Build history of the part. All positions in model axes, mm. Face numbers are marked on the shaded views. A direction names the side the tool comes from. Round coordinates to 2 decimals unless told otherwise and drop trailing zeros. Order: outer loops, then holes, each group sorted by start corner. A loop starts at its lowest first (then second) coordinate and runs counter-clockwise, first axis right, second up. Notation, with made-up numbers: (69, 63) - (125, 63) arc R31 cw to (125, 92) - close; hole circle Ø4 at (40.25, -17.75). An arc over 180 degrees is marked (long way). One line per question, with ' | ' between items. Start each with the question number.
from build123d import *

# Parameters (mm, degrees)
SKETCH1_R          = 5
EXTRUDE1_DEPTH     = 40
SKETCH2_W          = 7
SKETCH2_H          = 34.499518557
SKETCH2_W_2        = 12
CUT_EXTRUDE1_DEPTH = 40


with BuildPart() as part:
    # Sketch1 → Extrude1 (new body)
    with BuildSketch(Plane.XY):
        with BuildLine():
            Line((15, -16), (25, -16))
            Line((25, -16), (25, -22))
            Line((25, -22), (-25, -22))
            Line((-25, -22), (-25, -16))
            Line((-25, -16), (-15, -16))
            Line((-15, -16), (-15, 0))
            ThreePointArc((-15, 0), (0, 15), (15, 0))
            Line((15, 0), (15, -16))
        make_face()
        Circle(SKETCH1_R, mode=Mode.SUBTRACT)
    extrude(amount=EXTRUDE1_DEPTH)

    # Sketch2 → Cut-Extrude1 (cut)
    with BuildSketch(Plane(origin=(15, 0, 0), x_dir=(0, 0, -1), z_dir=(1, 0, 0))):
        with Locations((-36.5, 1.249759279)):
            Rectangle(SKETCH2_W, SKETCH2_H)
        with Locations((-3.5, 1.249759279)):
            Rectangle(SKETCH2_W, SKETCH2_H)
        with Locations((-20, 1.249759279)):
            Rectangle(SKETCH2_W_2, SKETCH2_H)
    extrude(amount=-CUT_EXTRUDE1_DEPTH, mode=Mode.SUBTRACT)


solid = part.part
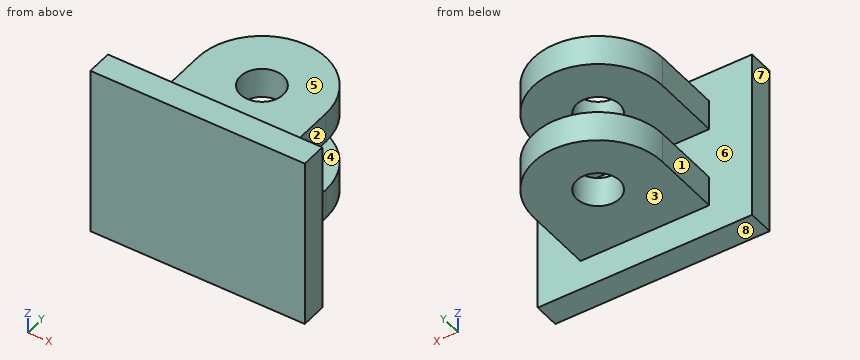
Item 1: Slice it at D-D (x = 6). Write the cut outline in (y, z).
Item 2: 3-axis set-ups, long thin cutter, end or side, ignore diameter. For the marked faces 1, 2, 3, 4 and 5: which of +Z, -Z, +X, -X, +Y, -Y reach the whole face in a straight line?
Item 3: Pull direction Z, two halves, no side cores. Call the marked faces 6, 7 and 8: released by +Z, released by -Z, zero draft, split by the parting line, or undercut.
Item 4: Pin check, flat tips, straight feed: pin 1 (9 mm diameter, centred on x = 4, y = 4, fed in from +Z); pin 2 (4 mm diameter, centred on x = 3, y = 8, fed in from -Z); pin 3 (3.5 mm diameter, centred on y = -9, z = 30, fed in from +X); pin 4 (6 mm diameter, centred on x = 0, y = 0, fed in from +Z). Stop position of each tip, or through.
Item 5: Wall check: line 1 along Y through (x, z) = (0, 31.75); line 2 along Z through (x, y) = (3, 6); line 3 along Y through (x, z) = (0, 4). Give the ranges that are in metal, low to high. Write a range as [from, to].
Item 6: Slice it at A-A (z = 10). Write the cut outline in (x, y), plus the area to 3 significant figures.
Item 7: Slice it at C-C (x = 0). Write the cut outline in (y, z).
Item 8: Slice it at B-B (y = -8). Write the cut outline in (x, z).
A:
1) outline: (-22, 0) - (-16, 0) - (-16, 7) - (13.75, 7) - (13.75, 14) - (-16, 14) - (-16, 26) - (13.75, 26) - (13.75, 33) - (-16, 33) - (-16, 40) - (-22, 40) - close
2) face 1: +Z, -Z, -X, +Y | face 2: +Z, -Z, +X, +Y | face 3: -Z, +X, -X, +Y | face 4: +X, -X, +Y | face 5: +Z, +X, -X, +Y
3) face 6: undercut | face 7: zero draft | face 8: released by -Z
4) pin 1: z = 33 | pin 2: z = 7 | pin 3: x = 15 | pin 4: through
5) line 1: [-22, -5], [5, 15] | line 2: [7, 14], [26, 33] | line 3: [-22, -16]
6) outline: (-25, -22) - (25, -22) - (25, -16) - (15, -16) - (15, 0) arc R15 ccw to (-15, 0) - (-15, -16) - (-25, -16) - close; hole circle Ø10 at (0, 0) | area: 1,050 mm^2
7) outline: (-22, 0) - (-16, 0) - (-16, 7) - (-5, 7) - (-5, 14) - (-16, 14) - (-16, 26) - (-5, 26) - (-5, 33) - (-16, 33) - (-16, 40) - (-22, 40) - close; (5, 7) - (15, 7) - (15, 14) - (5, 14) - close; (5, 26) - (15, 26) - (15, 33) - (5, 33) - close
8) outline: (-15, 7) - (15, 7) - (15, 14) - (-15, 14) - close; (-15, 26) - (15, 26) - (15, 33) - (-15, 33) - close
